Can you work these out from the model? Positions are in its coordinate system, mm. Coordinates: 2 decimals unless noted, no trailing zeros. Order: outer loops, then holes, each group sorted by start corner. A loop starts at its lowest first (then second) coordinate and runs counter-clockwise, first axis right, second up. Notation, with made-up numbers: (5.25, -40) -> (31.25, -40) arc R11 ccw to (31.25, -19) -> close; hole circle Ø9 at (-1.75, 32.25). An arc over 180 degrees is marked (long way). Write item = value, one per line.
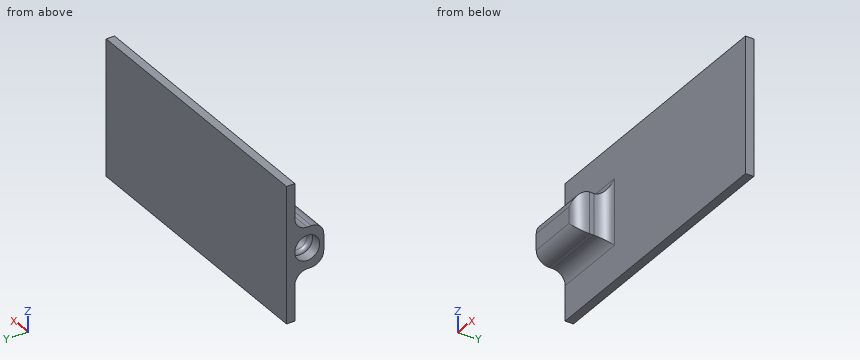
```python
from build123d import *

# Parameters (mm, degrees)
BOSS_EXTRUDE1_DEPTH      = 3
BOSS_EXTRUDE1_DEPTH_BACK = 4
SKETCH1_W                = 15
SKETCH1_H                = 10
SKETCH2_R                = 2.3
CUT_EXTRUDE3_DEPTH       = 10
SKETCH2_4_R              = 3.025
SKETCH2_4_R_2            = 2.3
CUT_EXTRUDE4_DEPTH       = 2.6
CUT_EXTRUDE5_START       = 6.44
SKETCH2_5_R              = 3.025
SKETCH2_5_R_2            = 2.3
CUT_EXTRUDE5_DEPTH       = 3.56
SKETCH3_W                = 66
SKETCH3_H                = 33
BOSS_EXTRUDE2_DEPTH      = 2
FILLET2_R                = 3
FILLET3_R                = 3


with BuildPart() as part:
    # Sketch1 → Boss-Extrude1 (new, two sides: drawn at the far end of the back side and taken through both)
    with BuildSketch(Plane(origin=(0, 0, 0), x_dir=(1, 0, 0), z_dir=(0, 1, 0)).offset(-BOSS_EXTRUDE1_DEPTH_BACK)):
        with Locations((7.5, 0)):
            Rectangle(SKETCH1_W, SKETCH1_H)
    extrude(amount=BOSS_EXTRUDE1_DEPTH + BOSS_EXTRUDE1_DEPTH_BACK)

    # Sketch2 → Cut-Extrude3 (cut)
    with BuildSketch(Plane(origin=(0, 0, 0), x_dir=(0, 0, -1), z_dir=(1, 0, 0))):
        Circle(SKETCH2_R)
    extrude(amount=CUT_EXTRUDE3_DEPTH, mode=Mode.SUBTRACT)

    # Sketch2<4> → Cut-Extrude4 (cut)
    with BuildSketch(Plane(origin=(0, 0, 0), x_dir=(0, 0, -1), z_dir=(1, 0, 0))):
        Circle(SKETCH2_4_R)
        Circle(SKETCH2_4_R_2, mode=Mode.SUBTRACT)
    extrude(amount=CUT_EXTRUDE4_DEPTH, mode=Mode.SUBTRACT)

    # Sketch2<5> → Cut-Extrude5 (cut)
    with BuildSketch(Plane(origin=(0, 0, 0), x_dir=(0, 0, -1), z_dir=(1, 0, 0)).offset(CUT_EXTRUDE5_START)):
        Circle(SKETCH2_5_R)
        Circle(SKETCH2_5_R_2, mode=Mode.SUBTRACT)
    extrude(amount=CUT_EXTRUDE5_DEPTH, mode=Mode.SUBTRACT)

    # Fillet1: read off the stored shape, not the designer's step
    # Fillet1 outline → Fillet1 (revolve, cut)
    with BuildSketch(Plane.YX):
        with BuildLine():
            Line((2.3, 2.6), (3.025000061, 2.599999982))
            ThreePointArc((3.025000061, 2.599999982), (2.501564048, 2.959364472), (2.3, 3.561444226))
            Line((2.3, 3.561444226), (2.3, 2.6))
        make_face()
    revolve(axis=Axis((0, 0, 0), (1, 0, 0)), mode=Mode.SUBTRACT)

    # Sketch3 → Boss-Extrude2 (add)
    with BuildSketch(Plane(origin=(0, 3, 0), x_dir=(1, 0, 0), z_dir=(0, 1, 0))):
        with Locations((33, 0)):
            Rectangle(SKETCH3_W, SKETCH3_H)
    extrude(amount=BOSS_EXTRUDE2_DEPTH)

    # Fillet2
    fillet2_edges = [part.edges().sort_by_distance(p)[0] for p in [
        (7.5, 3, 5),
        (15, 3, 0),
        (7.5, 3, -5),
    ]]
    fillet(fillet2_edges, radius=FILLET2_R)

    # Fillet3
    fillet3_edges = [part.edges().sort_by_distance(p)[0] for p in [
        (15, -4, 0),
        (7.5, -4, -5),
        (7.5, -4, 5),
    ]]
    fillet(fillet3_edges, radius=FILLET3_R)


solid = part.part
```
Item 1: I'm going to push flat-ended pins straight in: P1, Ø1.1, axis at y = -0.5, z = 1, coming from the +X side; P2, Ø3, axis at y = 1, z = -0.5, coming from the +X side; P3, Ø16.5, axis at x = 38.5, z = 7, coming from the -Y side. Where does each tip first touch, or does it pass through?
A:
P1 = 15
P2 = 16.34
P3 = 3
Item 2: If I drill on probe 1 along Y at (x, z) = (0.7, 0) (3 decimals); probe 2 along Y at (x, z) = (5.7, 0); probe 3 along Y at (x, z) = (18, -9.5), over which ranges is the centre line in solid material (lowest first)?
A:
probe_1 = -4 to -3.025, 3 to 5
probe_2 = -4 to -2.3, 2.3 to 5
probe_3 = 3 to 5
Item 3: I want a section at B-B, the plane x = 52. Please give me the cut outline in (y, z).
A:
outline = (3, -16.5) -> (5, -16.5) -> (5, 16.5) -> (3, 16.5) -> close
Item 4: I want a section at A-A, the plane z = 10. Please give me the cut outline in (x, y).
A:
outline = (0, 3) -> (66, 3) -> (66, 5) -> (0, 5) -> close
